from build123d import *

# Parameters (mm, degrees)
EXTRUDE_1_DEPTH = 2
MM_2_D          = 3
MM_3_D          = 3


with BuildPart() as part:
    # 草图2 → 凸台-拉伸1 (new body)
    with BuildSketch(Plane.XY):
        with BuildLine():
            Line((-50.360367403, 22.370399323), (9.639632597, 22.370399323))
            ThreePointArc((9.639632597, 22.370399323), (16.710700409, 19.441467134), (19.639632597, 12.370399323))
            Line((19.639632597, 12.370399323), (19.639632597, -2.629600677))
            ThreePointArc((19.639632597, -2.629600677), (16.710700409, -9.700668489), (9.639632597, -12.629600677))
            Line((9.639632597, -12.629600677), (-50.360367403, -12.629600677))
            ThreePointArc((-50.360367403, -12.629600677), (-57.431435215, -9.700668489), (-60.360367403, -2.629600677))
            Line((-60.360367403, -2.629600677), (-60.360367403, 12.370399323))
            ThreePointArc((-60.360367403, 12.370399323), (-57.431435215, 19.441467134), (-50.360367403, 22.370399323))
        make_face()
    extrude(amount=EXTRUDE_1_DEPTH)

    # 大小mm 暗销孔2 (through all)
    with Locations(Plane(origin=(-41.610367403, 13.620399323, 0), x_dir=(-1, 0, 0), z_dir=(0, 0, -1))):
        with Locations((0, 0), (8.75, 0), (0, -17.352577314), (8.75, -17.352577314)):
            Hole(MM_2_D / 2)

    # 大小mm 暗销孔3 (through all)
    with Locations(Plane(origin=(9.639632597, 13.620399323, 0), x_dir=(-1, 0, 0), z_dir=(0, 0, -1))):
        with Locations((0, 0), (8.75, 0), (8.75, -17.352577314), (0, -17.352577314)):
            Hole(MM_3_D / 2)


solid = part.part
Geometry check sheet. Reference: the model listing, model coordinates, mm. Round coordinates to 2 decimals unless told otherwise and drop trailing zeros. Order: outer loops, then holes, each group sorted by start corner. A loop starts at its lowest first (then second) coordinate and runs counter-clockwise, first axis right, second up. Notation, with made-up numbers: M 78.25,-6 L 90.25,-6 A29 cw 90.25,25 Z; hole C 24,59.5 d4. An arc over 180 degrees is marked long. Write each question's results on one line, items separated by ' | '. Start each with the question number.
1. Cross-section at C-C on y = 16. Record the boundary of the cut face in (x, z), plus the area to 3 significant figures.
2. Cross-section at B-B on x = -55. Record the boundary of the cut face in (y, z), plus the area to 3 significant figures.
3. Cross-section at A-A on z = 1.55. Give the number of separate pieces and of enclosed holes in the cut face, plus the area to 3 significant figures.
4. Material ranges on L1, parallel to Y at x = 0.5, z = 0.8; L2, parallel to Y at x = 0, z = 0.5; L3, parallel to X at y = -7.5, z = 1.6, recorded low to high. Write a range as from..to.
5. Draft check along X on faces 1 (the face through (19.64, 5, 1)), 2 (the face through (11.025, -4.307, 1.014)), 3 (the face through (-60.36, 5, 1)). Enter one of: pulls with the +X half, pulls with the -X half, needs draft (parallel to the pull), parting line crosses it, or undercut.
Resolved:
1) outline: M -59.68,0 L 18.96,0 L 18.96,2 L -59.68,2 Z | area: 157 mm2
2) outline: M -11.49,0 L 21.23,0 L 21.23,2 L -11.49,2 Z | area: 65.4 mm2
3) separate pieces: 1 | enclosed holes: 8 | area: 2,660 mm2
4) L1: -12.63..-5.18, -2.28..12.17, 15.07..22.37 | L2: -12.63..-4.94, -2.52..12.41, 14.83..22.37 | L3: -59.09..18.37
5) face 1: pulls with the +X half | face 2: undercut | face 3: pulls with the -X half
